```python
from build123d import *

# Parameters (mm, degrees)
F0_R        = 7
F1_DEPTH    = 91
F2_R        = 11
F3_T        = -3
F4_DEPTH    = 100
F5_T1_DEPTH = 5.6326126102
F5_T3_DEPTH = 5.6326126102


# Not quite as in the source:
# - a fillet or chamfer that OpenCascade refuses, or shapes differently, is made with other operations: its cross-section is extruded or revolved along the edge and cut away or added


with BuildPart() as f1:
    # F0 (on Right) → F1 (new body)
    with BuildSketch(Plane.YZ):
        with BuildLine():
            ThreePointArc((-5.1046863561, 14.1046863561), (8.6148042537, 12.2794603982), (15, 0))
            ThreePointArc((15, 0), (10.6066017178, -10.6066017178), (0, -15))
            Line((0, -15), (37, -15))
            Line((37, -15), (37, 25))
            Line((37, 25), (25, 25))
            Line((25, 25), (-5.1046863561, 14.1046863561))
        make_face()
        with BuildLine():
            ThreePointArc((0, -15), (10.6066017178, -10.6066017178), (15, 0))
            ThreePointArc((15, 0), (8.6148042537, 12.2794603982), (-5.1046863561, 14.1046863561))
            ThreePointArc((-5.1046863561, 14.1046863561), (-14.7744762232, -2.5913032105), (0, -15))
        make_face()
        Circle(F0_R, mode=Mode.SUBTRACT)
        Circle(F0_R)
    extrude(amount=-F1_DEPTH)

    # F2
    f2_edges = [f1.edges().sort_by_distance(p)[0] for p in [
        (0, 37, 5),
        (-91, 37, 5),
    ]]
    fillet(f2_edges, radius=F2_R)

    # F3
    f3_openings = [f1.faces().sort_by_distance(p)[0] for p in [
        (-45.5, -14.774476, -2.591303),
        (-45.5, 18.248672, -15),
        (-45.5, 9.947657, 19.552343),
        (-45.5, 30.82309, 25),
    ]]
    offset(amount=F3_T, openings=f3_openings)

    # F0 (on Right) → F4 (cut)
    with BuildSketch(Plane.YZ):
        Circle(F0_R)
    extrude(amount=-F4_DEPTH, mode=Mode.SUBTRACT)

    # F5: fillet of radius 3 on 4 edges, made by hand

    # F5_s2 → F5_t1 (cut)
    with BuildSketch(Plane.YZ.offset(-4.3163063051)):
        with BuildLine():
            ThreePointArc((25.5265223701, 25.0004), (25.0078471195, 24.9552591608), (24.504768349, 24.821194021))
            Line((24.504768349, 24.821194021), (24.4025929469, 25.1035134232))
            ThreePointArc((24.4025929469, 25.1035134232), (24.6502768349, 25.1927283501), (24.8978245979, 25.2823194021))
            Line((24.8978245979, 25.2823194021), (25, 25.30024))
            ThreePointArc((25, 25.30024), (25.263261185, 25.30024), (25.5265223701, 25.30064))
            Line((25.5265223701, 25.30064), (25.5265223701, 25.0004))
        make_face()
    extrude(amount=F5_T1_DEPTH, mode=Mode.SUBTRACT)

    # F5_s4 → F5_t3 (cut)
    with BuildSketch(Plane.YZ.offset(-92.3163063051)):
        with BuildLine():
            ThreePointArc((25.5265223701, 25.0004), (25.0078471195, 24.9552591608), (24.504768349, 24.821194021))
            Line((24.504768349, 24.821194021), (24.4025929469, 25.1035134232))
            ThreePointArc((24.4025929469, 25.1035134232), (24.6502768349, 25.1927283501), (24.8978245979, 25.2823194021))
            Line((24.8978245979, 25.2823194021), (25, 25.30024))
            ThreePointArc((25, 25.30024), (25.263261185, 25.30024), (25.5265223701, 25.30064))
            Line((25.5265223701, 25.30064), (25.5265223701, 25.0004))
        make_face()
    extrude(amount=F5_T3_DEPTH, mode=Mode.SUBTRACT)


solid = f1.part
```
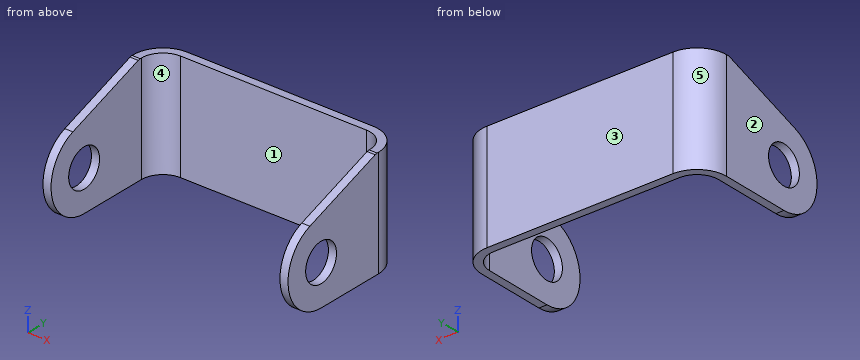
Work out the finished part from the listing and answer in its coordinate system (mm). Face numbers are marked on the shaded views. A direction names the side the tool comes from. Round coordinates to 2 decimals unless told otherwise and drop trailing zeros. Write each loop counter-clockwise with the first axis right and the second up, starting at its lowest first coordinate (ties: lowest second). Pieces come first, ordered by that corner, then holes. Notation, with made-up numbers: (0.25, 58) - (14.25, 58) arc R23 ccw to (14.25, 88) - close; hole circle Ø1 at (87.25, -6). An arc over 180 degrees is marked (long way). Return JSON: item names as keys, results as strings. Group by question number.
Q1. The part is cut by section B-B on y = 11.5. Write down the section's boundary in (x, z), then the cut area to 3 significant figures.
Q2. The part is cut by section A-A on z = 0. Write down the section's boundary in (x, y), then the cut area to 3 significant figures.
Q3. For the marked faces 1 and 2, determine the directions among +Z, -Z, +X, -X, +Y, -Y from which every point of the face is accessible in a straight line to the end or side of a thin tool.
Q4. The part is cut by section C-C on z = 18.5. Write down the section's boundary in (x, y), then the cut area to 3 significant figures.
Q5. Each of these flat-tipped pins is pushed along its axis until it touches: pin 1 Ø3 at (x, z) = (-23, -1.5) entering from -Y; pin 2 Ø4 at (y, z) = (-5.5, 16) entering from +X. Where does it stop, or does it pass through?
Q6. Find the intervals of material crossed by L1, parallel to X at y = 25, z = 8.5; L2, parallel to Y at x = -52, z = 13.5; L3, parallel to X at y = 28, z = -9, in increasing order.
Q7. The mould has two halves that part along X. Classify the marked faces 3, 4 and 5: released by +X, released by -X, zero draft, split by the parting line, or undercut.
Q8. The part is cut by section D-D on x = -60. Write down the section's boundary in (y, z).
Solved:
{
 "1": {"outline": "(-91, -15) - (-88, -15) - (-88, 20.11) - (-91, 20.11) - close; (-3, -15) - (0, -15) - (0, 20.11) - (-3, 20.11) - close", "area": "211 mm²"},
 "2": {"outline": "(-91, -15) - (-88, -15) - (-88, -7) - (-91, -7) - close; (-91, 7) - (-88, 7) - (-88, 26) arc R8 cw to (-80, 34) - (-11, 34) arc R8 cw to (-3, 26) - (-3, 7) - (0, 7) - (0, 26) arc R11 ccw to (-11, 37) - (-80, 37) arc R11 ccw to (-91, 26) - close; (-3, -15) - (0, -15) - (0, -7) - (-3, -7) - close", "area": "459 mm²"},
 "3": {"face 1": "+Z, -Z, -Y", "face 2": "+Z, -Z, -X, +Y, -Y"},
 "4": {"outline": "(-91, 7.04) - (-88, 7.04) - (-88, 26) arc R8 cw to (-80, 34) - (-11, 34) arc R8 cw to (-3, 26) - (-3, 7.04) - (0, 7.04) - (0, 26) arc R11 ccw to (-11, 37) - (-80, 37) arc R11 ccw to (-91, 26) - close", "area": "410 mm²"},
 "5": {"pin 1": "y = 34", "pin 2": "x = 0"},
 "6": {"L1": "-91 to -88, -3 to 0", "L2": "34 to 37", "L3": "-90.82 to -87.75, -3.25 to -0.18"},
 "7": {"face 3": "zero draft", "face 4": "undercut", "face 5": "released by -X"},
 "8": {"outline": "(34, -15) - (37, -15) - (37, 25) - (34, 25) - close"}
}
